```python
from build123d import *

# Parameters (mm, degrees)
SKETCH_R            = 88
SKETCH_R_2          = 6
PAD_DEPTH           = 4
SKETCH002_R         = 5
PAD001_DEPTH        = 18.5
POLARPATTERN_COUNT  = 3
SKETCH001_R         = 85
SKETCH001_R_2       = 56
PAD002_DEPTH        = 5
LINEARPATTERN_COUNT = 2
LINEARPATTERN_PITCH = 17


with BuildPart() as part:
    # Sketch → Pad (new body)
    with BuildSketch(Plane.XZ.offset(18.5)):
        Circle(SKETCH_R)
        Circle(SKETCH_R_2, mode=Mode.SUBTRACT)
        with BuildLine():
            ThreePointArc((9.369863, -75.420194), (65.817931, -38), (70.000735, 29.595558))
            ThreePointArc((70.000735, 29.595558), (68.191495, 31.271602), (65.737549, 31.025388))
            Line((19.522712, 4.34324), (65.737549, 31.025388))
            ThreePointArc((6, -19.078784), (17.320508, -10), (19.522712, 4.34324))
            Line((6, -19.078784), (6, -72.443081))
            ThreePointArc((6, -72.443081), (7.013746, -74.691368), (9.369863, -75.420194))
        make_face(mode=Mode.SUBTRACT)
        with BuildLine():
            Line((-6, -19.078784), (-6, -72.443081))
            ThreePointArc((-9.369863, -75.420194), (-7.013746, -74.691368), (-6, -72.443081))
            ThreePointArc((-70.000735, 29.595558), (-65.817931, -38), (-9.369863, -75.420194))
            ThreePointArc((-65.737549, 31.025388), (-68.191495, 31.271602), (-70.000735, 29.595558))
            Line((-65.737549, 31.025388), (-19.522712, 4.34324))
            ThreePointArc((-19.522712, 4.34324), (-17.320508, -10), (-6, -19.078784))
        make_face(mode=Mode.SUBTRACT)
        with BuildLine():
            Line((13.522712, 14.735544), (59.737549, 41.417693))
            ThreePointArc((59.737549, 41.417693), (61.177749, 43.419766), (60.630872, 45.824636))
            ThreePointArc((60.630872, 45.824636), (0, 76), (-60.630872, 45.824636))
            ThreePointArc((-60.630872, 45.824636), (-61.177749, 43.419766), (-59.737549, 41.417693))
            Line((-13.522712, 14.735544), (-59.737549, 41.417693))
            ThreePointArc((13.522712, 14.735544), (0, 20), (-13.522712, 14.735544))
        make_face(mode=Mode.SUBTRACT)
    pad = extrude(amount=PAD_DEPTH)

    # Sketch002 → Pad001 (join, symmetric)
    with BuildSketch(Plane.XZ):
        with Locations((0, -72.5)):
            Circle(SKETCH002_R)
    pad001 = extrude(amount=PAD001_DEPTH, both=True)

    # PolarPattern: Pad001 ×3 about axis
    polarpattern_axis = Axis((0, 0, 0), (0, -1, 0))
    for i in range(1, POLARPATTERN_COUNT):
        add(pad001.rotate(polarpattern_axis, i * 360 / POLARPATTERN_COUNT))

    # Sketch001 → Pad002 (join)
    with BuildSketch(Plane.XZ.offset(8)):
        Circle(SKETCH001_R)
        Circle(SKETCH001_R_2, mode=Mode.SUBTRACT)
        with BuildLine():
            ThreePointArc((9.355263, -78.444114), (68.416007, -39.5), (72.612227, 31.120162))
            ThreePointArc((72.612227, 31.120162), (70.801772, 32.785003), (68.354801, 32.536459))
            Line((54.701064, 24.653471), (68.354801, 32.536459))
            ThreePointArc((6, -59.699246), (51.961524, -30), (54.701064, 24.653471))
            Line((6, -59.699246), (6, -75.465224))
            ThreePointArc((6, -75.465224), (7.008241, -77.708635), (9.355263, -78.444114))
        make_face(mode=Mode.SUBTRACT)
        with BuildLine():
            Line((-6, -59.699246), (-6, -75.465224))
            ThreePointArc((-9.355263, -78.444114), (-7.008241, -77.708635), (-6, -75.465224))
            ThreePointArc((-72.612227, 31.120162), (-68.416007, -39.5), (-9.355263, -78.444114))
            ThreePointArc((-68.354801, 32.536459), (-70.801772, 32.785003), (-72.612227, 31.120162))
            Line((-68.354801, 32.536459), (-54.701064, 24.653471))
            ThreePointArc((-54.701064, 24.653471), (-51.961524, -30), (-6, -59.699246))
        make_face(mode=Mode.SUBTRACT)
        with BuildLine():
            Line((48.701064, 35.045776), (62.354801, 42.928764))
            ThreePointArc((62.354801, 42.928764), (63.793532, 44.923632), (63.256964, 47.323953))
            ThreePointArc((63.256964, 47.323953), (0, 79), (-63.256964, 47.323953))
            ThreePointArc((-63.256964, 47.323953), (-63.793532, 44.923632), (-62.354801, 42.928764))
            Line((-48.701064, 35.045776), (-62.354801, 42.928764))
            ThreePointArc((48.701064, 35.045776), (0, 60), (-48.701064, 35.045776))
        make_face(mode=Mode.SUBTRACT)
    pad002 = extrude(amount=PAD002_DEPTH)

    # LinearPattern: Pad002 ×2
    with Locations(*[(0, i * LINEARPATTERN_PITCH, 0) for i in range(1, LINEARPATTERN_COUNT)]):
        add(pad002)

    # Mirrored: Pad across XZ
    add(pad.mirror(Plane.XZ))


solid = part.part
```
The listing builds one solid part. Answer for the finished solid, in the listing's coordinates (mm). A direction names the side the tool comes from. Coordinates: 2 decimals unless noted, no trailing zeros. Write each loop counter-clockwise with the first axis right and the second up, starting at its lowest first coordinate (ties: lowest second). Pieces come first, ordered by that corner, then holes. Notation, with made-up numbers: (-29.75, 21.5) - (-7.75, 21.5) arc R19 ccw to (-7.75, 33.5) - close; hole circle Ø10 at (13.25, 6). An arc over 180 degrees is marked (long way). Return JSON: item names as keys, results as strings. Group by question number.
1. A cutting plane is placed at C-C, the plane y = 14. Determine the outline of the cut face in (x, z), plus the area to 3 significant figures.
2. Determine the mould class of faces 1 (the cylindrical face through (67.556, -2.084, 37.752)), 2 (the flat face through (42.31, -20.47, 17.5)), 3 (the cylindrical face through (-67.453, -10.465, -51.721)) for opening direction X: released by +X, released by -X, zero draft, split by the parting line, or undercut.
3. Given pin 1 (3 mm diameter, centred on y = 20.5, z = -48.5, fed in from +X); pin 2 (5 mm diameter, centred on x = 4, y = -1, fed in from +Z); pin 3 (2 mm diameter, centred on x = -17.5, y = 7, fed in from -Z); pin 4 (15.5 mm diameter, centred on x = 0, z = 0, fed in from +Y), each flat-ended and moving along its own axis, determine where each tip first touches the part or whether it passes through.
4. Straight lines are drawn through the part: L1, parallel to Z at x = 0, y = 5.9; L2, parallel to Y at x = -70, z = -51; L3, parallel to Y at x = 60, z = -59. For each, find the intervals that lie inside material, in ascending order.
5. Which of the six approach directions +Z, -Z, +X, -X, +Y, -Y give full straight-line access (tool end or side, diameter ignored) to faces 4 (the cylindrical face through (17.216, -20.472, -10.18)), 5 (the cylindrical face through (-67.78, -15.79, 36.47))?
6. A cutting plane is placed at A-A, the plane x = 0. Give the number of separate pieces and of enclosed holes in the cut face, plus the area to 3 significant figures.
Ans:
{
 "1": {"outline": "circle Ø10 at (-62.79, 36.25); circle Ø10 at (0, -72.5); circle Ø10 at (62.79, 36.25)", "area": "236 mm²"},
 "2": {"face 1": "undercut", "face 2": "undercut", "face 3": "split by the parting line"},
 "3": {"pin 1": "x = 74.4", "pin 2": "z = -67.73", "pin 3": "z = -83.38", "pin 4": "y = 22.5"},
 "4": {"L1": "-85 to -56, 56 to 60, 79 to 85", "L2": "-22.5 to -18.5, 18.5 to 22.5", "L3": "-22.5 to -18.5, -13 to -8, 4 to 9, 18.5 to 22.5"},
 "5": {"face 4": "+Y, -Y", "face 5": "none"},
 "6": {"separate pieces": "9", "enclosed holes": "0", "area": "1,520 mm²"}
}
